Autodesk Inventor part; units mm, degrees
ref_plane "YZ Plane" through (0, 0, 0) normal (1, 0, 0) x (0, 1, 0)
ref_plane "XZ Plane" through (0, 0, 0) normal (0, 1, 0) x (-1, 0, 0)
ref_plane "XY Plane" through (0, 0, 0) normal (0, 0, 1) x (1, 0, 0)
sketch "Boceto1" plane through (0, 0, 0) normal (0, 0, 1) x (1, 0, 0)
  line L0 (-26.5284, 23.7303) -> (2.6646, 23.7303)
  line L1 (-6.5284, -16.2697) -> (-26.5284, -16.2697)
  line L2 (-26.5284, -16.2697) -> (-26.5284, 23.7303)
  line L3 (-26.5284, 23.7303) -> (-6.5284, 23.7303)
  line L4 (-6.5284, 23.7303) -> (-6.5284, -16.2697)
  line L5 (-6.5284, -16.2697) -> (-26.5284, -16.2697)
  line L6 (-26.5284, -16.2697) -> (-26.5284, 23.7303)
  circle A0 centre (-16.5284, 13.7303) radius 3.15
  circle A1 centre (-16.5284, -6.2697) radius 3.15
  circle A2 centre (-16.5284, -6.2697) radius 5.05
  circle A3 centre (-16.5284, 13.7303) radius 5.0326
  line L7 (-6.5284, 23.7303) -> (-1.9384, 23.7303)
  circle A4 centre (-1.9384, 16.2303) radius 2
  line L8 (-6.5284, 23.7303) -> (2.6646, 23.7303)
  line L9 (2.6646, 23.7303) -> (2.6646, -11.2697)
  line L10 (2.6646, -11.2697) -> (-6.5284, -11.2697)
  line L11 (-6.5284, -11.2697) -> (-6.5284, 23.7303)
  circle A5 centre (-1.9319, -3.7697) radius 2
  circle A6 centre (-1.9319, -3.7697) radius 4.05
  circle A7 centre (-1.9384, 16.2303) radius 4.05
  point P0 (0, 0)
  point P1 (13.9631, 1.0984)
  point P2 (-16.5284, 23.7303)
  dimension "d0" = 6.3
  dimension "d1" = 6.3
  dimension "d2" = 10
  dimension "d3" = 10
  dimension "d4" = 10.1
  dimension "d5" = 4.59
  dimension "d6" = 4
  dimension "d7" = 7.5
  dimension "d8" = 35
  dimension "d9" = 4
  dimension "d10" = 7.5
  dimension "d11" = 8.1
  dimension "d12" = 8.1
extrude "Extrusión1" add sketch "Boceto1" along normal blind 3 contours L0 L4 L1 L2 | L0 L9 L10 L4
sketch "Boceto2" plane through (0, 0, 0) normal (0, 0, -1) x (-1, 0, 0)
  point P0 (0, 0)
sketch "Boceto3" plane through (0, 0, 3) normal (0, 0, 1) x (1, 0, 0)
  circle A0 centre (-1.9384, 16.2303) radius 4.05
  circle A1 centre (-1.9384, 16.2303) radius 2
  circle A2 centre (-1.9319, -3.7697) radius 4.05
  circle A3 centre (-1.9319, -3.7697) radius 2
  circle A4 centre (-16.5284, -6.2697) radius 5.05
  circle A5 centre (-16.5284, -6.2697) radius 3.15
  circle A6 centre (-16.5284, 13.7303) radius 5.0326
  circle A7 centre (-16.5284, 13.7303) radius 3.15
  point P0 (0, 0)
  dimension "d15" = 4
  dimension "d16" = 4
  dimension "d17" = 6.3
  dimension "d18" = 6.3
extrude "Extrusión2" add sketch "Boceto3" against normal blind 1.5 contours A0 | A2
extrude "Extrusión3" add sketch "Boceto3" against normal blind 6 contours A4 | A6
properties part number "Base Rodamiento delgado"
The model under review builds one solid part; all positions refer to its coordinate system, in mm. A direction names the side the tool comes from. Coordinates: 2 decimals unless noted, no trailing zeros. Write each loop counter-clockwise with the first axis right and the second up, starting at its lowest first coordinate (ties: lowest second). Pieces come first, ordered by that corner, then holes.
1) Machinability: for faces 1 (the face through (-4, 15, 1.5)), 2 (the face through (-26.528, 3, 1)), which of the approach directions +Z, -Z, +X, -X, +Y, -Y give a long, thin tool a straight path to every point of the face, cutting with its end or side? Answer none if there is none.
2) We need section A-A on x = -3. State the section outline as (y, z) points, then the cut area to 3 significant figures.
3) We need section C-C on z = -2.4. State the section outline as (x, y) points.
4) Clearance check with flat-ended pins moving along their axes: pin 1 Ø0.9 at (y, z) = (-14, 2) entering from +X; pin 2 Ø1.5 at (x, y) = (-1, 4) entering from -Z; pin 3 Ø3.5 at (x, z) = (-1, 1.5) entering from -Y. State where each tip first meets the part, or that it passes through.
5) We need section D-D on x = -8.75. State the section outline as (y, z) points.
6) We need section B-B on y = -4.5. State the section outline as (x, z) points.
7) To check wall thickness, follow probe 1 along Y at (x, z) = (-15.75, 2.7); probe 2 along Y at (x, z) = (-1, 0.55); probe 3 along Y at (x, z) = (-18.5, -1.7). State the ranges of each line that lie inside material, in increasing order.
8) The part is to be moulded in two halves that separate along Y. For faces 3 (the face through (-2, -11.27, 1)), 4 (the face through (-6.528, -14, 1)), 5 (the face through (-4, -5, 1.5)), say which applies: pulls with the +Y half, pulls with the -Y half, needs draft (parallel to the pull), parting line crosses it, or undercut.
Answer list:
1. face 1: -Z
1. face 2: +Z, -Z, -X, +Y, -Y
2. outline: (-11.27, 0) - (-7.68, 0) - (-7.68, 1.5) - (-5.46, 1.5) - (-5.46, 3) - (-11.27, 3) - close; (-2.08, 1.5) - (0.14, 1.5) - (0.14, 0) - (12.32, 0) - (12.32, 1.5) - (14.54, 1.5) - (14.54, 3) - (-2.08, 3) - close; (17.93, 1.5) - (20.14, 1.5) - (20.14, 0) - (23.73, 0) - (23.73, 3) - (17.93, 3) - close
2. area: 71.4 mm2
3. outline: circle Ø10.1 at (-16.53, -6.27); circle Ø10.07 at (-16.53, 13.73); hole circle Ø6.3 at (-16.53, -6.27); hole circle Ø6.3 at (-16.53, 13.73)
4. pin 1: stops at x = -6.53
4. pin 2: stops at z = 0
4. pin 3: stops at y = -11.27
5. outline: (-16.27, 0) - (23.73, 0) - (23.73, 3) - (-16.27, 3) - close
6. outline: (-26.53, 0) - (-21.26, 0) - (-21.26, -3) - (-19.13, -3) - (-19.13, 3) - (-26.53, 3) - close; (-13.92, -3) - (-11.8, -3) - (-11.8, 0) - (-5.92, 0) - (-5.92, 1.5) - (-3.79, 1.5) - (-3.79, 3) - (-13.92, 3) - close; (-0.07, 1.5) - (2.05, 1.5) - (2.05, 0) - (2.66, 0) - (2.66, 3) - (-0.07, 3) - close
7. probe 1: y = -16.27 to -9.32, -3.22 to 10.68, 16.78 to 23.73
7. probe 2: y = -11.27 to -7.71, 0.17 to 12.29, 20.17 to 23.73
7. probe 3: y = -10.92 to -8.73, -3.81 to -1.62, 9.1 to 11.27, 16.19 to 18.36
8. face 3: pulls with the -Y half
8. face 4: needs draft
8. face 5: undercut
